```python
from build123d import *

# Parameters (mm, degrees)
SKETCH2_R           = 1.224840395
BOSS_EXTRUDE1_DEPTH = 1.6


with BuildPart() as part:
    # Sketch2 → Boss-Extrude1 (new body)
    # profile 1 of 12: a face of its own
    with BuildSketch(Plane.XY):
        with BuildLine():
            ThreePointArc((-8.135, -17.059653426), (-4.170284778, -18.434172747), (0, -18.9))
            Line((0, -18.9), (0, -16.415))
            ThreePointArc((0, -16.415), (-2.059106624, -16.285340184), (-4.08568405, -15.898409066))
            ThreePointArc((-4.08568405, -15.898409066), (-5.118317114, -15.09992037), (-5.247629689, -13.801000241))
            ThreePointArc((-5.247629689, -13.801000241), (-8.401661187, -12.141553208), (-11.06618513, -9.774700592))
            Line((-11.06618513, -9.774700592), (-8.135, -17.059653426))
        make_face()
    # profile 2 of 12: a face of its own
    with BuildSketch(Plane.XY):
        with BuildLine():
            Line((0, -16.415), (0, -18.9))
            ThreePointArc((0, -18.9), (4.170284778, -18.434172747), (8.135, -17.059653426))
            Line((8.135, -17.059653426), (11.06618513, -9.774700592))
            ThreePointArc((11.06618513, -9.774700592), (8.401661187, -12.141553208), (5.247629689, -13.801000241))
            ThreePointArc((5.247629689, -13.801000241), (5.118317114, -15.09992037), (4.08568405, -15.898409066))
            ThreePointArc((4.08568405, -15.898409066), (2.059106624, -16.285340184), (0, -16.415))
        make_face()
    # profile 3 of 12: a face of its own
    with BuildSketch(Plane.XY):
        with BuildLine():
            ThreePointArc((5.247629689, -13.801000241), (8.401661187, -12.141553208), (11.06618513, -9.774700592))
            Line((11.06618513, -9.774700592), (12.90921384, -5.194172026))
            ThreePointArc((12.90921384, -5.194172026), (9.679242267, -9.996974249), (4.774656023, -13.070190697))
            ThreePointArc((4.774656023, -13.070190697), (5.060206981, -13.403841589), (5.247629689, -13.801000241))
        make_face()
    # profile 4 of 12: a face of its own
    with BuildSketch(Plane.XY):
        with BuildLine():
            Line((-12.909213852, -5.194171995), (-11.06618513, -9.774700592))
            ThreePointArc((-11.06618513, -9.774700592), (-8.401661187, -12.141553208), (-5.247629689, -13.801000241))
            ThreePointArc((-5.247629689, -13.801000241), (-5.060206981, -13.403841589), (-4.774656023, -13.070190697))
            ThreePointArc((-4.774656023, -13.070190697), (-9.679242279, -9.996974238), (-12.909213852, -5.194171995))
        make_face()
    # profile 5 of 12: a face of its own
    with BuildSketch(Plane.XY):
        with BuildLine():
            ThreePointArc((-12.909213987, 5.194171661), (-13.915, -1.8e-07), (-12.909213852, -5.194171995))
            ThreePointArc((-12.909213852, -5.194171995), (-9.679242279, -9.996974238), (-4.774656023, -13.070190697))
            ThreePointArc((-4.774656023, -13.070190697), (-4.065529678, -12.697217895), (-3.26431595, -12.702262254))
            ThreePointArc((-3.26431595, -12.702262254), (-1.64515281, -13.011406428), (0, -13.115))
            Line((0, -13.115), (0, -10.854127302))
            ThreePointArc((0, -10.854127302), (-10.854127302, 0), (0, 10.854127302))
            Line((0, 10.854127302), (0, 13.115))
            ThreePointArc((0, 13.115), (-1.64515281, 13.011406428), (-3.26431595, 12.702262254))
            ThreePointArc((-3.26431595, 12.702262254), (-4.065529678, 12.697217895), (-4.774656023, 13.070190697))
            ThreePointArc((-4.774656023, 13.070190697), (-9.679242408, 9.996974112), (-12.909213987, 5.194171661))
        make_face()
    # profile 6 of 12: a face of its own
    with BuildSketch(Plane.XY):
        with BuildLine():
            Line((-11.06618513, 9.774700592), (-12.909213987, 5.194171661))
            ThreePointArc((-12.909213987, 5.194171661), (-9.679242408, 9.996974112), (-4.774656023, 13.070190697))
            ThreePointArc((-4.774656023, 13.070190697), (-5.060206981, 13.403841589), (-5.247629689, 13.801000241))
            ThreePointArc((-5.247629689, 13.801000241), (-8.401661187, 12.141553208), (-11.06618513, 9.774700592))
        make_face()
    # profile 7 of 12: a face of its own
    with BuildSketch(Plane.XY):
        with BuildLine():
            Line((-8.135, 17.059653426), (-11.06618513, 9.774700592))
            ThreePointArc((-11.06618513, 9.774700592), (-8.401661187, 12.141553208), (-5.247629689, 13.801000241))
            ThreePointArc((-5.247629689, 13.801000241), (-5.118317114, 15.09992037), (-4.08568405, 15.898409066))
            ThreePointArc((-4.08568405, 15.898409066), (-2.059106624, 16.285340184), (0, 16.415))
            Line((0, 16.415), (0, 18.9))
            ThreePointArc((0, 18.9), (-4.170284778, 18.434172747), (-8.135, 17.059653426))
        make_face()
    # profile 8 of 12: a face of its own
    with BuildSketch(Plane.XY):
        with BuildLine():
            ThreePointArc((4.774656023, 13.070190697), (9.679242519, 9.996974005), (12.909214102, 5.194171376))
            Line((12.909214102, 5.194171376), (11.06618513, 9.774700592))
            ThreePointArc((11.06618513, 9.774700592), (8.401661187, 12.141553208), (5.247629689, 13.801000241))
            ThreePointArc((5.247629689, 13.801000241), (5.060206981, 13.403841589), (4.774656023, 13.070190697))
        make_face()
    # profile 9 of 12: a face of its own
    with BuildSketch(Plane.XY):
        with BuildLine():
            ThreePointArc((4.774656023, -13.070190697), (9.679242267, -9.996974249), (12.90921384, -5.194172026))
            ThreePointArc((12.90921384, -5.194172026), (13.661239614, -2.645327429), (13.915, 0))
            ThreePointArc((13.915, 0), (13.661239681, 2.645327085), (12.909214102, 5.194171376))
            ThreePointArc((12.909214102, 5.194171376), (9.679242519, 9.996974005), (4.774656023, 13.070190697))
            ThreePointArc((4.774656023, 13.070190697), (4.065529678, 12.697217895), (3.26431595, 12.702262254))
            ThreePointArc((3.26431595, 12.702262254), (1.64515281, 13.011406428), (0, 13.115))
            Line((0, 13.115), (0, 10.854127302))
            ThreePointArc((0, 10.854127302), (7.675027019, 7.675027019), (10.854127302, 0))
            ThreePointArc((10.854127302, 0), (7.675027019, -7.675027019), (0, -10.854127302))
            Line((0, -10.854127302), (0, -13.115))
            ThreePointArc((0, -13.115), (1.64515281, -13.011406428), (3.26431595, -12.702262254))
            ThreePointArc((3.26431595, -12.702262254), (4.065529678, -12.697217895), (4.774656023, -13.070190697))
        make_face()
    # profile 10 of 12: a face of its own
    with BuildSketch(Plane.XY):
        with BuildLine():
            ThreePointArc((5.247629689, 13.801000241), (8.401661187, 12.141553208), (11.06618513, 9.774700592))
            Line((11.06618513, 9.774700592), (8.135, 17.059653426))
            ThreePointArc((8.135, 17.059653426), (4.170284778, 18.434172747), (0, 18.9))
            Line((0, 18.9), (0, 16.415))
            ThreePointArc((0, 16.415), (2.059106624, 16.285340184), (4.08568405, 15.898409066))
            ThreePointArc((4.08568405, 15.898409066), (5.118317114, 15.09992037), (5.247629689, 13.801000241))
        make_face()
    # profile 11 of 12: a face of its own
    with BuildSketch(Plane.XY):
        with BuildLine():
            ThreePointArc((0, 10.854127302), (-10.854127302, 0), (0, -10.854127302))
            Line((0, -10.854127302), (0, -6.103787969))
            ThreePointArc((0, -6.103787969), (-6.103787969, 0), (0, 6.103787969))
            Line((0, 6.103787969), (0, 10.854127302))
        make_face()
        with Locations((-7.476059495, 0)):
            Circle(SKETCH2_R, mode=Mode.SUBTRACT)
    # profile 12 of 12: a face of its own
    with BuildSketch(Plane.XY):
        with BuildLine():
            Line((0, -6.103787969), (0, -10.854127302))
            ThreePointArc((0, -10.854127302), (7.675027019, -7.675027019), (10.854127302, 0))
            ThreePointArc((10.854127302, 0), (7.675027019, 7.675027019), (0, 10.854127302))
            Line((0, 10.854127302), (0, 6.103787969))
            ThreePointArc((0, 6.103787969), (4.316029864, 4.316029864), (6.103787969, 0))
            ThreePointArc((6.103787969, 0), (4.316029864, -4.316029864), (0, -6.103787969))
        make_face()
        with Locations((3.72330191, -6.482938258)):
            Circle(SKETCH2_R, mode=Mode.SUBTRACT)
        with Locations((7.476059495, 0)):
            Circle(SKETCH2_R, mode=Mode.SUBTRACT)
        with Locations((3.708670732, 6.491319355)):
            Circle(SKETCH2_R, mode=Mode.SUBTRACT)
    extrude(amount=BOSS_EXTRUDE1_DEPTH)


solid = part.part
```
Model file for the job. Use its own axes, mm. Give positions to 0.01 mm unless a question says otherwise; leave off trailing zeros. Write each loop counter-clockwise with the first axis right and the second up, starting at its lowest first coordinate (ties: lowest second). Pieces come first, ordered by that corner, then holes. Notation, with made-up numbers: (-13, 32) -> (21, 32) arc R12 ccw to (21, 40) -> close; hole circle Ø1 at (53.25, -2.5). An arc over 180 degrees is marked (long way). Use CSV: the item, a comma, the result in double quotes. Start each with the question number.
1) Cut at A-A on x = 11.5. List the corners of the cut face in (y, z).
2) Cut at C-C on z = 1.3. List the corners of the cut face in (x, y) (3 decimals).
3) Pin check, flat tip, straight feed: P1, Ø2, axis at x = 3.72, y = -6.48, coming from the -Z side. Stop position of the tip, or through.
4) Drill centre lines: L1, parallel to Y at x = 3, z = 0.85; L2, parallel to Y at x = -4.75, z = 0.95; L3, parallel to Y at x = 5, z = 1. Where is each one in solid material? Low to high.
5) Cut at B-B on y = -10.5. List the corners of the cut face in (x, z), plus the area to 3 significant figures.
6) Two-plate mould, pull along Y, no slides. Class faces 1 (the cylindrical face through (-13.915, 0.075, 0.789)), 2 (the flat face through (6, -4, 1.6)), 3 (the cylindrical face through (2.821, -5.655, 0.789)): released by +Y, released by -Y, zero draft, split by the parting line, or undercut.
Final values:
1,outline,"(-8.7, 0) -> (8.7, 0) -> (8.7, 1.6) -> (-8.7, 1.6) -> close"
2,outline,"(-12.909, -5.194) -> (-8.135, -17.06) arc R18.9 ccw to (8.135, -17.06) -> (12.909, -5.194) arc R13.915 ccw to (12.909, 5.194) -> (8.135, 17.06) arc R18.9 ccw to (-8.135, 17.06) -> (-12.909, 5.194) arc R13.915 ccw to start; hole circle Ø2.45 at (-7.476, 0); hole circle Ø12.208 at (0, 0); hole (-4.086, -15.898) arc R16.415 ccw to (4.086, -15.898) arc R1.65 ccw to (3.264, -12.702) arc R13.115 cw to (-3.264, -12.702) arc R1.65 ccw to start; hole (-4.086, 15.898) arc R1.65 ccw to (-3.264, 12.702) arc R13.115 cw to (3.264, 12.702) arc R1.65 ccw to (4.086, 15.898) arc R16.415 ccw to start; hole circle Ø2.45 at (3.709, 6.491); hole circle Ø2.45 at (3.723, -6.483); hole circle Ø2.45 at (7.476, 0)"
3,P1,"passes through"
4,L1,"y = -18.66 to -16.14, -12.77 to -7.47, -5.49 to -5.32, 5.32 to 5.49, 7.49 to 12.77, 16.14 to 18.66"
4,L2,"y = -18.29 to -15.55, -13.05 to -3.83, 3.83 to 13.05, 15.55 to 18.29"
4,L3,"y = -18.23 to -15.28, -13.32 to -3.5, 3.5 to 13.32, 15.28 to 18.23"
5,outline,"(-10.77, 0) -> (10.77, 0) -> (10.77, 1.6) -> (-10.77, 1.6) -> close"
5,area,"34.5 mm2"
6,face 1,"split by the parting line"
6,face 2,"zero draft"
6,face 3,"undercut"
